The listing builds one solid part. Answer for the finished solid, in the listing's coordinates (mm). Face numbers are marked on the shaded views. A direction names the side the tool comes from. Round coordinates to 2 decimals unless told otherwise and drop trailing zeros. Write each loop counter-clockwise with the first axis right and the second up, starting at its lowest first coordinate (ties: lowest second). Pieces come first, ordered by that corner, then holes. Notation, with made-up numbers: M 14.25,87.25 L 49.25,87.25 A17 ccw 49.25,92.25 Z; hole C -34.75,50.5 d5. An arc over 180 degrees is marked long. One line per item, written item: value. Start each with the question number.
(1) Section C-C (x = -1) is taken. Determine the outline of the cut face in (y, z).
(2) For the marked faces 3 and 4, determine the directions among +Z, -Z, +X, -X, +Y, -Y from which every point of the face is accessible in a straight line to the end or side of a thin tool.
(3) For a pull along X with two mould halves and no side action, classify the marked faces 1 and 2 as released by +X, released by -X, zero draft, split by the parting line, or undercut.
(4) Section A-A (x = -4.5) is taken. Determine the outline of the cut face in (y, z).
(5) Section B-B (z = 0.7) is taken. Determine the outline of the cut face in (x, y), plus the area to 3 significant figures.
(6) Section D-D (x = 9) is taken. Determine the outline of the cut face in (y, z).
(7) Given P1, Ø1, axis at x = -3.5, z = 1, coming from the +Y side; P2, Ø1, axis at x = -8.5, z = 1, coming from the -Y side; P3, Ø1, axis at y = -9.5, z = 0.5, coming from the +X side, each flat-ended and moving along its own axis, determine where each tip first touches the part or whether it passes through.
(8) Consider probe 1 along Y at (x, z) = (0.5, 1.7); probe 2 along Y at (x, z) = (-8, 1.25); probe 3 along X at (y, z) = (-10, 1.7). Determine where each line is inside the solid, lowest interval first.
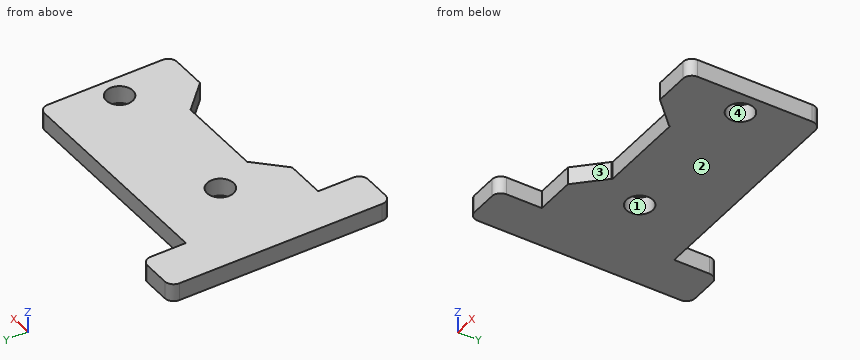
```python
from build123d import *

# Parameters (mm, degrees)
SKETCH1_R           = 1.5
BOSS_EXTRUDE1_DEPTH = 2


with BuildPart() as part:
    # Sketch1 → Boss-Extrude1 (new body)
    with BuildSketch(Plane.XY):
        with BuildLine():
            Line((-10.646329578, -7.696708369), (-10.646329578, -11.696708369))
            ThreePointArc((-10.646329578, -11.696708369), (-10.939222796, -12.40381515), (-11.646329578, -12.696708369))
            Line((-11.646329578, -12.696708369), (-14.646329578, -12.696708369))
            ThreePointArc((-14.646329578, -12.696708369), (-15.353436359, -12.40381515), (-15.646329578, -11.696708369))
            Line((-15.646329578, -11.696708369), (-15.646329578, 11.303291631))
            ThreePointArc((-15.646329578, 11.303291631), (-15.353436359, 12.010398412), (-14.646329578, 12.303291631))
            Line((-14.646329578, 12.303291631), (-11.646329578, 12.303291631))
            ThreePointArc((-11.646329578, 12.303291631), (-10.939222796, 12.010398412), (-10.646329578, 11.303291631))
            Line((-10.646329578, 11.303291631), (-10.646329578, 7.303291631))
            Line((-10.646329578, 7.303291631), (13.863670422, 7.303291631))
            ThreePointArc((13.863670422, 7.303291631), (14.570777204, 7.010398412), (14.863670422, 6.303291631))
            Line((14.863670422, 6.303291631), (14.863670422, -6.696708369))
            ThreePointArc((14.863670422, -6.696708369), (14.570777204, -7.40381515), (13.863670422, -7.696708369))
            Line((13.863670422, -7.696708369), (9.863670422, -7.696708369))
            Line((9.863670422, -7.696708369), (6.863670422, -4.696708369))
            Line((6.863670422, -4.696708369), (6.863670422, -4.605403467))
            Line((6.863670422, -4.605403467), (-3.136329578, -4.605403467))
            Line((-3.136329578, -4.605403467), (-3.136329578, -4.696708369))
            Line((-3.136329578, -4.696708369), (-6.136329578, -7.696708369))
            Line((-6.136329578, -7.696708369), (-10.646329578, -7.696708369))
        make_face()
        with Locations((12.353670422, -0.196708369)):
            Circle(SKETCH1_R, mode=Mode.SUBTRACT)
        with Locations((-5.146329578, -0.196708369)):
            Circle(SKETCH1_R, mode=Mode.SUBTRACT)
    extrude(amount=BOSS_EXTRUDE1_DEPTH)


solid = part.part
```
Recorded:
1. outline: M -4.61,0 L 7.3,0 L 7.3,2 L -4.61,2 Z
2. face 3: +Z, -Z, -Y
2. face 4: +Z, -Z
3. face 1: undercut
3. face 2: zero draft
4. outline: M -6.06,0 L -1.55,0 L -1.55,2 L -6.06,2 Z; M 1.16,0 L 7.3,0 L 7.3,2 L 1.16,2 Z
5. outline: M -15.65,-11.7 A1 ccw -14.65,-12.7 L -11.65,-12.7 A1 ccw -10.65,-11.7 L -10.65,-7.7 L -6.14,-7.7 L -3.14,-4.7 L -3.14,-4.61 L 6.86,-4.61 L 6.86,-4.7 L 9.86,-7.7 L 13.86,-7.7 A1 ccw 14.86,-6.7 L 14.86,6.3 A1 ccw 13.86,7.3 L -10.65,7.3 L -10.65,11.3 A1 ccw -11.65,12.3 L -14.65,12.3 A1 ccw -15.65,11.3 Z; hole C -5.15,-0.2 d3; hole C 12.35,-0.2 d3
5. area: 452 mm2
6. outline: M -6.83,0 L 7.3,0 L 7.3,2 L -6.83,2 Z
7. P1: stops at y = 7.3
7. P2: stops at y = -7.7
7. P3: stops at x = -10.65
8. probe 1: y = -4.61 to 7.3
8. probe 2: y = -7.7 to 7.3
8. probe 3: x = -15.65 to -10.65
